Input: part model. Units: mm. Frame: model coordinates. Face numbers are marked on the shaded views. A direction names the side the tool comes from. Coordinates: 2 decimals unless noted, no trailing zeros. Loops run counter-clockwise (first coordinate to the right, second up) from the corner with the lowest first, then second, coordinate; pieces in that order, holes last. Notation, with made-up numbers: M -23,1.25 L 4,1.25 A33 ccw 4,39.25 Z; hole C 85.5,-30 d6. An arc over 180 degrees is marked long. Use a Markdown table: item, result. Add a question column.
1. Section C-C on y = 3. Output: boundary loops of the cut face in (x, z), then the cut area to 3 significant figures.
2. Draft query along Z for the marked faces 1, 2 and 3. Return one class per face: +Z half, -Z half, draft (parallel to the pull), parting line (faces both ways), or undercut.
3. Set-up query: the marked faces 4 and 5. Return all of +Z, -Z, +X, -X, +Y, -Y with unobstructed straight access to the full face (end or side cutting, diameter ignored); none if empty.
4. Pin query (flat end, axial travel): pin 1 (4.5 mm diameter, centred on x = 12.37, z = 12.37, fed in from +Y); pin 2 (4 mm diameter, centred on x = 7, y = 6, fed in from -Z); pin 3 (1.6 mm diameter, centred on y = 0.5, z = -1.5, fed in from -X); pin 4 (0.6 mm diameter, centred on y = 1.5, z = 0.5, fed in from +X). Return the tip coordinate at first contact, or that it passes through.
5. Section D-D on x = 7.5. Output: boundary loops of the cut face in (y, z), then the cut area to 3 significant figures.
6. Section A-A on z = 0. Output: boundary loops of the cut face in (x, y).
7. Line query: L1, parallel to X at y = 6, z = 13; L2, parallel to Z at x = 12, y = 3; L3, parallel to X at y = 4.5, z = 0. Output: solid intervals per line, ascending. Write a range as [from, to].
8. Section B-B on x = 0. Output: boundary loops of the cut face in (y, z).
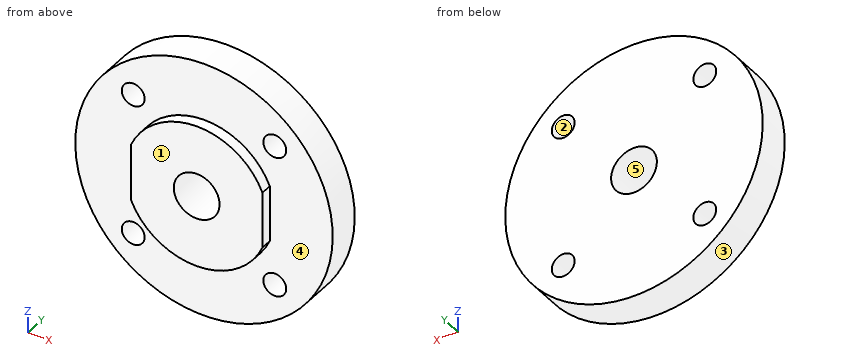
```python
from build123d import *

# Parameters (mm, degrees)
BIT_ATTACHED_TO_SHAFT_DEPTH = 2
SKETCH2_R                   = 22.5
BOSS_EXTRUDE2_DEPTH         = 6
SKETCH3_R                   = 2
CUT_EXTRUDE1_DEPTH          = 6
SKETCH4_R                   = 4
CUT_EXTRUDE2_DEPTH          = 33.810059433


with BuildPart() as part:
    # Sketch1 → bit attached to shaft (new body)
    with BuildSketch(Plane(origin=(0, 0, 0), x_dir=(1, 0, 0), z_dir=(0, 1, 0))):
        with BuildLine():
            Line((11.5, -4.898979486), (11.5, 4.898979486))
            ThreePointArc((11.5, 4.898979486), (0, 12.5), (-11.5, 4.898979486))
            Line((-11.5, 4.898979486), (-11.5, -4.898979486))
            ThreePointArc((-11.5, -4.898979486), (0, -12.5), (11.5, -4.898979486))
        make_face()
    extrude(amount=BIT_ATTACHED_TO_SHAFT_DEPTH)

    # Sketch2 → Boss-Extrude2 (add)
    with BuildSketch(Plane(origin=(0, 2, 0), x_dir=(1, 0, 0), z_dir=(0, 1, 0))):
        with Locations(Location((0, 0, 0), (0, 0, 270))):
            Circle(SKETCH2_R)
    extrude(amount=BOSS_EXTRUDE2_DEPTH)

    # Sketch3 → Cut-Extrude1 (cut)
    with BuildSketch(Plane.XZ.offset(-2)):
        with Locations(Location((-12.374368671, -12.374368671, 0), (0, 0, 270))):
            Circle(SKETCH3_R)
        with Locations(Location((12.374368671, -12.374368671, 0), (0, 0, 270))):
            Circle(SKETCH3_R)
        with Locations(Location((12.374368671, 12.374368671, 0), (0, 0, 270))):
            Circle(SKETCH3_R)
        with Locations(Location((-12.374368671, 12.374368671, 0), (0, 0, 270))):
            Circle(SKETCH3_R)
    extrude(amount=-CUT_EXTRUDE1_DEPTH, mode=Mode.SUBTRACT)

    # Sketch4 → Cut-Extrude2 (cut, through all)
    with BuildSketch(Plane.XZ):
        with Locations(Location((0, 0, 0), (0, 0, 270))):
            Circle(SKETCH4_R)
    extrude(amount=-CUT_EXTRUDE2_DEPTH, mode=Mode.SUBTRACT)


solid = part.part
```
Answers below:
| question | item | result |
|---|---|---|
| 1 | outline | C 0,0 d45; hole C -12.37,-12.37 d4; hole C -12.37,12.37 d4; hole C 0,0 d8; hole C 12.37,-12.37 d4; hole C 12.37,12.37 d4 |
| 1 | area | 1,490 mm² |
| 2 | face 1 | draft |
| 2 | face 2 | undercut |
| 2 | face 3 | parting line |
| 3 | face 4 | -Y |
| 3 | face 5 | +Y, -Y |
| 4 | pin 1 | stops at y = 8 |
| 4 | pin 2 | stops at z = -21.94 |
| 4 | pin 3 | stops at x = -11.5 |
| 4 | pin 4 | stops at x = 11.5 |
| 5 | outline | M 0,-10 L 2,-10 L 2,-21.21 L 8,-21.21 L 8,21.21 L 2,21.21 L 2,10 L 0,10 Z |
| 5 | area | 295 mm² |
| 6 | outline | M -22.5,2 L -11.5,2 L -11.5,0 L -4,0 L -4,8 L -22.5,8 Z; M 4,0 L 11.5,0 L 11.5,2 L 22.5,2 L 22.5,8 L 4,8 Z |
| 7 | L1 | x = [-18.36, -14.27], [-10.47, 10.47], [14.27, 18.36] |
| 7 | L2 | z = [-19.03, -14.34], [-10.41, 10.41], [14.34, 19.03] |
| 7 | L3 | x = [-22.5, -4], [4, 22.5] |
| 8 | outline | M 0,-12.5 L 2,-12.5 L 2,-22.5 L 8,-22.5 L 8,-4 L 0,-4 Z; M 0,4 L 8,4 L 8,22.5 L 2,22.5 L 2,12.5 L 0,12.5 Z |
